Geometry check sheet. Reference: the model listing, model coordinates, mm. A direction names the side the tool comes from. Round coordinates to 2 decimals unless told otherwise and drop trailing zeros. Loops run counter-clockwise (first coordinate to the right, second up) from the corner with the lowest first, then second, coordinate; pieces in that order, holes last. Notation, with made-up numbers: M 4,82.25 L 9,82.25 A30 ccw 9,112.25 Z; hole C 30,-15.5 d5. An arc over 180 degrees is marked long. Write item = value, one per line.
from build123d import *

# Parameters (mm, degrees)
SKETCH1_W           = 38
SKETCH1_H           = 20
BOSS_EXTRUDE1_DEPTH = 2
SKETCH2_W           = 5
SKETCH2_H           = 20
BOSS_EXTRUDE2_DEPTH = 7
M3_TAPPED_HOLE1_D   = 2.5
SKETCH7_R           = 1.15
CUT_EXTRUDE1_DEPTH  = 7.5
CUT_EXTRUDE2_DEPTH  = 7.5
SKETCH9_W           = 5
SKETCH9_H           = 20
BOSS_EXTRUDE3_DEPTH = 2.5
FILLET1_R           = 2
CHAMFER1_SIZE       = 0.9


with BuildPart() as part:
    # Sketch1 → Boss-Extrude1 (new body)
    with BuildSketch(Plane.XY):
        with Locations((19, 10)):
            Rectangle(SKETCH1_W, SKETCH1_H)
    extrude(amount=BOSS_EXTRUDE1_DEPTH)

    # Sketch2 → Boss-Extrude2 (add)
    with BuildSketch(Plane.XY.offset(2)):
        with Locations((-2.5, 10)):
            Rectangle(SKETCH2_W, SKETCH2_H)
    extrude(amount=-BOSS_EXTRUDE2_DEPTH)

    # M3 Tapped Hole1 (through all)
    with Locations(Plane(origin=(-5, 10, -2.5), x_dir=(0, -1, 0), z_dir=(-1, 0, 0))):
        with Locations((0, 0)):
            Hole(M3_TAPPED_HOLE1_D / 2)

    # Sketch7 → Cut-Extrude1 (cut)
    with BuildSketch(Plane.XY.offset(2)):
        with Locations((35, 17.75)):
            Circle(SKETCH7_R)
        with Locations((5, 17.75)):
            Circle(SKETCH7_R)
        with Locations((35, 2.25)):
            Circle(SKETCH7_R)
        with Locations((5, 2.25)):
            Circle(SKETCH7_R)
    extrude(amount=-CUT_EXTRUDE1_DEPTH, mode=Mode.SUBTRACT)

    # Sketch8 → Cut-Extrude2 (cut)
    with BuildSketch(Plane.XY.offset(2)):
        with BuildLine():
            Line((30, 4.25), (10, 4.25))
            ThreePointArc((10, 4.25), (4.25, 10), (10, 15.75))
            Line((10, 15.75), (30, 15.75))
            ThreePointArc((30, 15.75), (35.75, 10), (30, 4.25))
        make_face()
    extrude(amount=-CUT_EXTRUDE2_DEPTH, mode=Mode.SUBTRACT)

    # Sketch9 → Boss-Extrude3 (add)
    with BuildSketch(Plane(origin=(0, 0, -5), x_dir=(-1, 0, 0), z_dir=(0, 0, -1))):
        with Locations((2.5, 10)):
            Rectangle(SKETCH9_W, SKETCH9_H)
    extrude(amount=BOSS_EXTRUDE3_DEPTH)

    # Fillet1
    fillet1_edges = [part.edges().sort_by_distance(p)[0] for p in [
        (38, 20, 1),
        (38, 0, 1),
    ]]
    fillet(fillet1_edges, radius=FILLET1_R)

    # Chamfer1
    chamfer1_edges = [part.edges().sort_by_distance(p)[0] for p in [
        (3.85, 17.75, 2),
        (33.85, 2.25, 2),
        (3.85, 2.25, 2),
        (33.85, 17.75, 2),
    ]]
    chamfer(chamfer1_edges, length=CHAMFER1_SIZE)


solid = part.part
(1) Sectioned sample at A-A on y = 10. Record the cut outline in (x, z), then the cut area to 3 significant figures.
Result set:
outline = M -5,-7.5 L 0,-7.5 L 0,-3.75 L -5,-3.75 Z; M -5,-1.25 L 0,-1.25 L 0,0 L 4.25,0 L 4.25,2 L -5,2 Z; M 35.75,0 L 38,0 L 38,2 L 35.75,2 Z
area = 48.0 mm2
(2) Sectioned sample at C-C on x = 10.5. Record the cut outline in (y, z).
Result set:
outline = M 0,0 L 4.25,0 L 4.25,2 L 0,2 Z; M 15.75,0 L 20,0 L 20,2 L 15.75,2 Z
(3) Tool access check on faces 4 (the flat face through (-2, 10, -7.5)), 5 (the flat face through (19, 3, 0)), 6 (the flat face through (20, 4.25, 1)). Record the directions out of +Z, -Z, +X, -X, +Y, -Y that give a thin tool (end or side, any length) a straight path to the whole face; none if there is none.
Result set:
face_4 = -Z, +X, -X, +Y, -Y
face_5 = -Z, +X, +Y, -Y
face_6 = +Z, -Z
(4) Depth check by flat-ended pin: pin 1 Ø3 at (x, y) = (5, 2.25) entering from +Z; pin 2 Ø3 at (x, y) = (35, 17.75) entering from -Z; pin 3 Ø3 at (y, z) = (2.5, -6) entering from +X. Enter the tip coordinate at first touch or a pass-through.
Result set:
pin_1 = 1.45
pin_2 = 0
pin_3 = 0
(5) Material ranges on line 1 along Y through (x, z) = (35, 0.25); line 2 along X through (y, z) = (1.5, -2.5); line 3 along Z through (x, y) = (1, 8), recorded low to high. Write a range as from..to.
Result set:
line_1 = 0..1.1, 3.4..7.16, 12.84..16.6, 18.9..20
line_2 = -5..0
line_3 = 0..2
(6) Release check for a two-part mould opening along Y. For faces 1 (the flat face through (20, 15.75, 1)), 2 (the flat face through (38, 10, 1)), 3 (the cylindrical face through (37.43, 0.6, 1.01)) record: released by +Y, released by -Y, zero draft, split by the parting line, or undercut.
Result set:
face_1 = undercut
face_2 = zero draft
face_3 = released by -Y
(7) Sectioned sample at B-B on z = -2.5. Record the cut outline in (x, y).
Result set:
outline = M -5,0 L 0,0 L 0,8.75 L -5,8.75 Z; M -5,11.25 L 0,11.25 L 0,20 L -5,20 Z
(8) Sectioned sample at D-D on z = 0.5. Record the cut outline in (x, y), then the cut area to 3 significant figures.
Result set:
outline = M -5,0 L 36,0 A2 ccw 38,2 L 38,18 A2 ccw 36,20 L -5,20 Z; hole C 5,2.25 d2.3; hole C 5,17.75 d2.3; hole M 10,4.25 L 30,4.25 A5.75 ccw 30,15.75 L 10,15.75 A5.75 ccw Z; hole C 35,2.25 d2.3; hole C 35,17.75 d2.3
area = 508 mm2
